Geometry: final body of the model. Coordinates: model frame, mm. Face numbers are marked on the shaded views. A direction names the side the tool comes from. Give positions to 0.01 mm unless a question says otherwise; leave off trailing zeros. Write each loop counter-clockwise with the first axis right and the second up, starting at its lowest first coordinate (ties: lowest second). Pieces come first, ordered by that corner, then holes. Notation, with made-up numbers: M -39.5,85 L -22.5,85 A13 cw -22.5,91 Z; hole C -5,-1.75 d6. An arc over 180 degrees is marked long. Use a Markdown table: item, result. Add a question column.
1) Pin query (flat end, axial travel): pin 1 (3 mm diameter, centred on x = 34.5, z = 40, fed in from +Y); pin 2 (10 mm diameter, centred on x = 1, y = 0, fed in from +Z); pin 3 (3 mm diameter, centred on x = 51.5, y = -20, fed in from +Z). Return the tip coordinate at first contact, or that it passes through.
2) Set-up query: the marked faces 1, 2, 3 and 4. Return all of +Z, -Z, +X, -X, +Y, -Y with unobstructed straight access to the full face (end or side cutting, diameter ignored); none if empty.
3) Line query: line 1 (Y direction, x = 14, z = 22.5); line 2 (Z direction, x = 4.5, y = 56.5) (3 decimals); line 3 (Z direction, x = 92, y = 19) (3 decimals). Output: solid intervals per line, ascending.
4) Section B-B on y = -34. Return the cut outline in (x, z) (3 decimals), then the cut area to 3 significant figures.
5) Draft query along X for the marked faces 5, 6, 7 and 8. Return one class per face: +X half, -X half, draft (parallel to the pull), parting line (faces both ways), or undercut.
6) Section A-A on x = 83. Return the cut outline in (y, z) (3 decimals).
```python
from build123d import *

# Parameters (mm, degrees)
F1_DEPTH = 63.5
F2_DEPTH = 25.4
F3_DEPTH = 25.4
F4_DEPTH = 7.9375
F0_W     = 25.4
F0_H     = 4.7498
F6_R     = 6.35


with BuildPart() as f1:
    # F0 (on Front) → F1 (new body, symmetric)
    with BuildSketch(Plane.XZ):
        Polygon((41.275, -9.525), (41.275, 9.525), (22.225, 9.525), (-41.275, 9.525), (-41.275, -9.525), align=None)
    extrude(amount=F1_DEPTH, both=True)

    # F0 (on Front) → F2 (join, symmetric)
    with BuildSketch(Plane.XZ):
        with BuildLine():
            Line((22.225, 9.525), (41.275, 9.525))
            Line((41.275, 9.525), (41.275, 27.0002))
            ThreePointArc((41.275, 27.0002), (45.9246798487, 38.2255201513), (57.15, 42.8752))
            Line((57.15, 42.8752), (60.325, 42.8752))
            Line((60.325, 42.8752), (60.325, 61.9252))
            Line((60.325, 61.9252), (57.15, 61.9252))
            add(Edge.make_bspline(
                [(55.6799774515, 61.8942490443), (56.1687606706, 61.9057674523), (56.6587732076, 61.9160843441), (57.15, 61.9252)],
                knots=[110.5461106931, 110.5461106931, 110.5461106931, 110.5461106931, 111.5045361635, 111.5045361635, 111.5045361635, 111.5045361635], degree=3))
            ThreePointArc((55.6799774515, 61.8942490443), (31.9399210383, 51.1705856764), (22.225, 27.0002))
            Line((22.225, 27.0002), (22.225, 9.525))
        make_face()
    extrude(amount=F2_DEPTH, both=True)

    # F0 (on Front) → F3 (join, symmetric)
    with BuildSketch(Plane.XZ):
        Polygon((60.325, 61.9252), (60.325, 42.8752), (85.725, 42.8752), (85.725, 52.3875), (85.725, 61.9252), align=None)
    extrude(amount=F3_DEPTH, both=True)

    # F0 (on Front) → F4 (join, symmetric)
    with BuildSketch(Plane.XZ):
        with BuildLine():
            Line((-41.275, 9.525), (22.225, 9.525))
            Line((22.225, 9.525), (22.225, 27.0002))
            ThreePointArc((22.225, 27.0002), (31.9399210383, 51.1705856764), (55.6799774515, 61.8942490443))
            add(Edge.make_bspline(
                [(-41.275, 9.525), (-40.7194862303, 43.2526218667), (-0.696950661, 60.5657000443), (55.6799774515, 61.8942490443)],
                knots=[0, 0, 0, 0, 110.5461106931, 110.5461106931, 110.5461106931, 110.5461106931], degree=3))
        make_face()
    extrude(amount=F4_DEPTH, both=True)

    # F0 (on Front) → F5 (revolve)
    with BuildSketch(Plane.XZ):
        Polygon((85.725, 52.3875), (85.725, 42.8752), (85.725, 38.1), (111.125, 38.1), (111.125, 61.9252), (85.725, 61.9252), align=None)
        with Locations((98.425, 64.3001)):
            Rectangle(F0_W, F0_H)
    revolve(axis=Axis((85.725, 0, 45.24375), (0, 0, 1)))

    # F6
    f6_edges = [f1.edges().sort_by_distance(p)[0] for p in [
        (-41.275, 63.5, 0),
        (-41.275, -63.5, 0),
        (41.275, -63.5, 0),
        (41.275, 63.5, 0),
    ]]
    fillet(f6_edges, radius=F6_R)


solid = f1.part
```
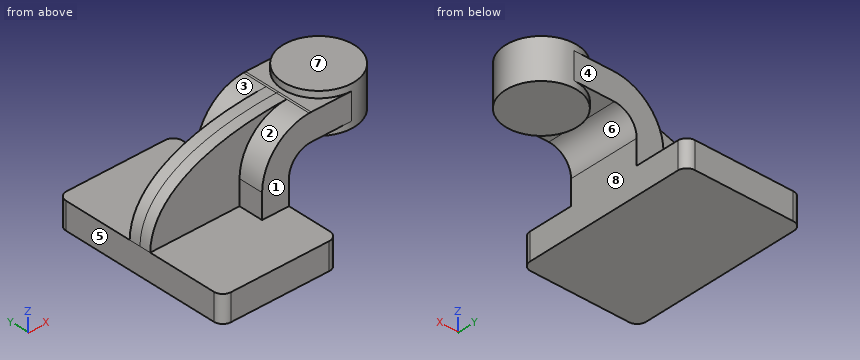
Found:
| question | item | result |
|---|---|---|
| 1 | pin 1 | y = 25.4 |
| 1 | pin 2 | z = 55.33 |
| 1 | pin 3 | z = 61.68 |
| 2 | face 1 | +Z, +X, -X, -Y |
| 2 | face 2 | +Z, -X, -Y |
| 2 | face 3 | +Z, -X, +Y |
| 2 | face 4 | +Z, +X, -X, +Y |
| 3 | line 1 | -7.94 to 7.94 |
| 3 | line 2 | -9.525 to 9.525 |
| 3 | line 3 | 38.1 to 66.675 |
| 4 | outline | M -41.275,-9.525 L 41.275,-9.525 L 41.275,9.525 L -41.275,9.525 Z |
| 4 | area | 1,570 mm² |
| 5 | face 5 | -X half |
| 5 | face 6 | undercut |
| 5 | face 7 | draft |
| 5 | face 8 | +X half |
| 6 | outline | M -25.4,42.875 L -25.253,42.875 L -25.253,38.1 L 25.253,38.1 L 25.253,42.875 L 25.4,42.875 L 25.4,61.925 L 25.253,61.925 L 25.253,66.675 L -25.253,66.675 L -25.253,61.925 L -25.4,61.925 Z |
